Source: CAD feature listing. Evaluate the final solid. Frame: model axes, mm. A direction names the side the tool comes from. Round coordinates to 2 decimals unless told otherwise and drop trailing zeros. Write each loop counter-clockwise with the first axis right and the second up, starting at its lowest first coordinate (ties: lowest second). Pieces come first, ordered by that corner, then holes. Notation, with made-up numbers: M 25.5,0 L 52.5,0 A20 ccw 52.5,15 Z; hole C 44.25,8 d7. An arc over 180 degrees is marked long. Answer in a Markdown table with one row per item. Add a question column.
Item 1: Contact query for flat-ended pins moving along their axis: pin 1 (21 mm diameter, centred on y = 20, z = 292.5, fed in from +X); pin 2 (13 mm diameter, centred on x = 24.5, z = 338, fed in from +Y); pin 3 (5 mm diameter, centred on x = 13, y = 5.5, fed in from +Z). Output: stop coordinate, or through.
Item 2: Set-up query: faces 1 (the face through (12, 4, 12)), 2 (the face through (4.762, 23, 276)). Return all of +Z, -Z, +X, -X, +Y, -Y with unobstructed straight access to the full face (end or side cutting, diameter ignored); none if empty.
Item 3: Material intervals for probe 1 along Y at (x, z) = (18, 314); probe 2 along Z at (x, y) = (2.5, 29), sorted ascending.
Item 4: Cut plane C-C on y = 23. Return loops of the section in (x, z).
Item 5: Cut plane A-A on z = 506. Return loops of the section in (x, y), and give its area (3 significant figures).
Item 6: Cut plane B-B on x = 21.5. Return loops of the section in (y, z), and give its area (3 significant figures).
Autodesk Inventor part; units mm, degrees
ref_plane "Start plane" through (0, 0, 0) normal (0, 0, 1) x (1, 0, 0)
ref_plane "End plane" through (0, 0, 558.8) normal (0, 0, 1) x (1, 0, 0)
ref_plane "Work Plane4" through (0, 19.05, 558.8) normal (0.7071, 0, 0.7071) x (0.7071, 0, -0.7071)
ref_plane "Start plane" through (0, 0, 0) normal (0, 0, 1) x (1, 0, 0)
ref_plane "End plane" through (0, 0, 558.8) normal (0, 0, 1) x (1, 0, 0)
sketch "Sketch" plane through (0, 0, 0) normal (0, 0, 1) x (1, 0, 0)
  line L0 (38.1, 0) -> (0, 0)
  line L1 (0, 0) -> (0, 38.1)
  line L2 (0, 38.1) -> (2.4765, 38.1)
  line L3 (4.7625, 35.814) -> (4.7625, 9.5885)
  line L4 (9.5885, 4.7625) -> (35.814, 4.7625)
  line L5 (38.1, 2.4765) -> (38.1, 0)
  line L6 (0, -11.0414) -> (0, 31.5385) construction
  line L7 (-11.0414, 0) -> (31.5385, 0) construction
  arc A0 (4.7625, 9.5885) -> (9.5885, 4.7625) centre (9.5885, 9.5885) ccw
  arc A1 (4.7625, 35.814) -> (2.4765, 38.1) centre (2.4765, 35.814) ccw
  arc A2 (38.1, 2.4765) -> (35.814, 4.7625) centre (35.814, 2.4765) ccw
  line L8 (0, 48.4964) -> (0, -20.9644) construction
  line L9 (-20.9644, 0) -> (48.4964, 0) construction
  point P0 (4.7625, 38.1)
  point P1 (4.7625, 4.7625)
  point P2 (38.1, 4.7625)
  dimension "d0" = 38.1
  dimension "d1" = 38.1
  dimension "d2" = 4.7625
  dimension "d3" = 4.7625
  dimension "d10" = 0
  dimension "d11" = 0
  dimension "d14" = 4.826
  dimension "d15" = 2.286
extrude "Body" add sketch "Sketch" along normal up to surface (558.8 mm away) from surface at 0
sketch "Sketch3" plane through (0, 0, 0) normal (0, 0, 1) x (1, 0, 0)
  line L0 (0, 0) -> (10, 0)
ref_plane "Work Plane3" through (0, 0, 0) normal (0, -1, 0) x (1, 0, 0)
sketch "Sketch4" plane through (0, 0, 0) normal (0, -1, 0) x (1, 0, 0)
  line L0 (-2, 0) -> (12, 0)
  line L1 (-2, 558.8) -> (12, 558.8)
  dimension "d17" = 558.8
ref_plane "Work Plane4" through (0, 19.05, 558.8) normal (0.7071, 0, 0.7071) x (0.7071, 0, -0.7071)
split "Split1" plane through (0, 19.05, 558.8) removes the side toward (0.7071, 0, 0.7071)
ref_plane "Work Plane5" through (0, 19.05, 0) normal (0.7071, 0, -0.7071) x (-0.7071, 0, -0.7071)
split "Split2" plane through (0, 19.05, 0) removes the side toward (0.7071, 0, -0.7071)
equation "\"d0\" = G_H"
equation "\"d1\" = G_H"
equation "\"d2\" = G_T"
equation "\"d3\" = G_T"
equation "\"d14\" = G_IR"
equation "\"d15\" = G_ER"
equation "\"d4\" = G_L"
equation "\"G_H\" = 38.1"
equation "\"G_T\" = 4.7625"
equation "\"G_ER\" = 2.286"
equation "\"G_IR\" = 4.826"
equation "\"G_L\" = d17"
equation "\"ex\" = 0"
equation "\"G_OFFSET_START\" = 0"
equation "\"G_OFFSET_END\" = 0"
equation "\"d13\" = G_OFFSET_END + B_L"
equation "\"B_L\" = 558.8"
properties part number "AISC - L 1.5 x 1.5 x 3/16 - 22" material "Aluminum 6061"
Results below:
| question | item | result |
|---|---|---|
| 1 | pin 1 | x = 4.76 |
| 1 | pin 2 | y = 4.76 |
| 1 | pin 3 | z = 548.19 |
| 2 | face 1 | -Z, +X, +Y, -Y |
| 2 | face 2 | +Z, -Z, +X, +Y |
| 3 | probe 1 | 0 to 4.76 |
| 3 | probe 2 | 2.5 to 556.3 |
| 4 | outline | M 0,0 L 4.76,4.76 L 4.76,554.04 L 0,558.8 Z |
| 5 | outline | M 0,0 L 38.1,0 L 38.1,2.48 A2.29 ccw 35.81,4.76 L 9.59,4.76 A4.83 cw 4.76,9.59 L 4.76,35.81 A2.29 ccw 2.48,38.1 L 0,38.1 Z |
| 5 | area | 343 mm2 |
| 6 | outline | M 0,21.5 L 4.76,21.5 L 4.76,537.3 L 0,537.3 Z |
| 6 | area | 2,460 mm2 |
